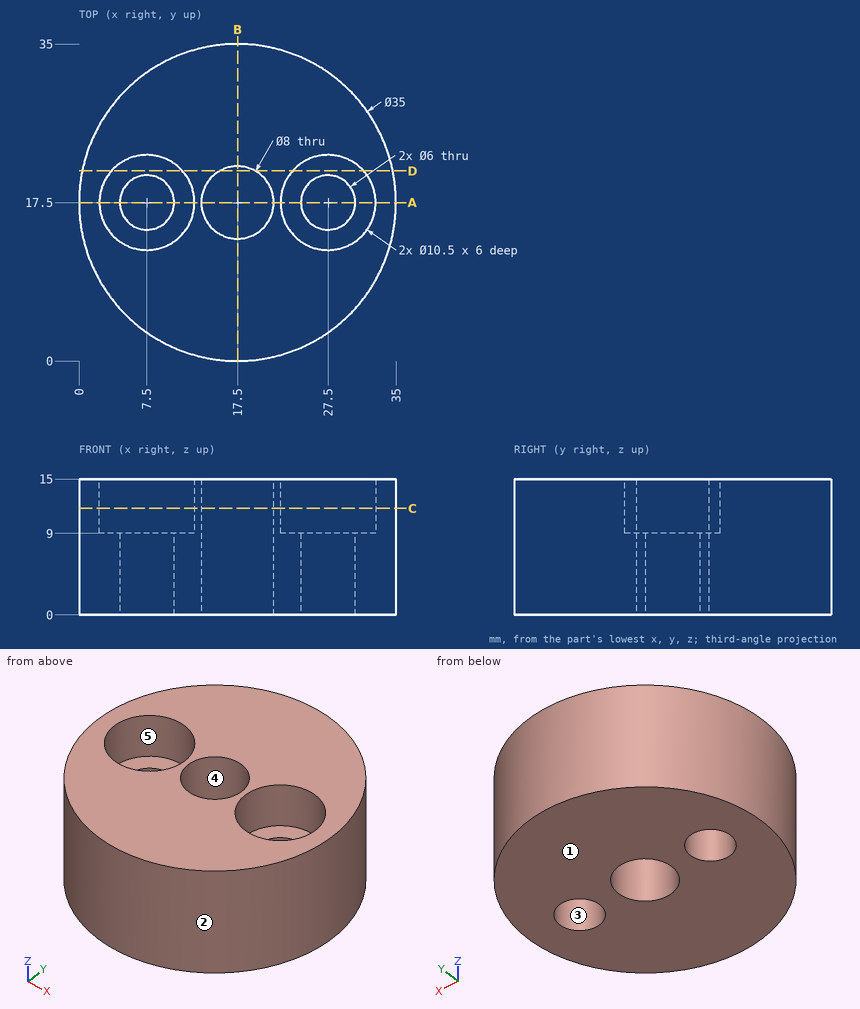
For this review, use the dimensioned drawing (mm, ordinates from the lowest corner) and the shaded views. A direction names the side the tool comes from. Give positions to 0.01 mm unless a question says otherwise; leave off trailing zeros. Order: outer loops, then holes, each group sorted by start corner. A loop starts at its lowest first (then second) coordinate and runs counter-clockwise, first axis right, second up. Notation, with made-up numbers: (6, -24) - (52, -24) arc R20 ccw to (52, 2) - close; hole circle Ø1 at (25, 37.25). An arc over 180 degrees is marked (long way). Use CSV: the item, a comma, the result in double quotes. Start each with the question number.
Q1. We need section B-B, the plane x = 17.5. Write out the cut boundary in (y, z), and give its area (3 significant figures).
Q2. We need section A-A, the plane y = 17.5. Write out the cut boundary in (x, z).
Q3. Tool access review of the marked faces 4 and 5: name each direction out of +Z, -Z, +X, -X, +Y, -Y from which nothing blocks a thin tool from reaching the whole face with its end or side.
Q4. To check wall thickness, follow line 1 along X through (y, z) = (15, 13); line 2 along Z through (x, y) = (24, 14.5); line 3 along Y through (x, z) = (7, 8.5). State the ranges of each line that lie inside material, in increasing order. Write a range as [from, to].
Q5. Clearance check with flat-ended pins moving along their axes: pin 1 Ø8 at (x, y) = (16, 17) entering from -Z; pin 2 Ø8 at (x, y) = (27.5, 17.5) entering from +Z; pin 3 Ø1 at (y, z) = (13.5, 3.5) entering from -X; pin 4 Ø2 at (y, z) = (21.5, 9) entering from -X. State where each tip first meets the part, or that it passes through.
Q6. We need section C-C, the plane z = 11.75. Write out the cut boundary in (x, y).
Q7. We need section D-D, the plane y = 21. Write out the cut boundary in (x, z), and give its area (3 significant figures).
Q8. The part is to be moulded in two halves that separate along Y. For the marked faces 1, 2 and 3, say which applies: +Y half, -Y half, draft (parallel to the pull), parting line (faces both ways), or undercut.
Outcome:
1,outline,"(0, 0) - (13.5, 0) - (13.5, 15) - (0, 15) - close; (21.5, 0) - (35, 0) - (35, 15) - (21.5, 15) - close"
1,area,"405 mm^2"
2,outline,"(0, 0) - (4.5, 0) - (4.5, 9) - (2.25, 9) - (2.25, 15) - (0, 15) - close; (10.5, 0) - (13.5, 0) - (13.5, 15) - (12.75, 15) - (12.75, 9) - (10.5, 9) - close; (21.5, 0) - (24.5, 0) - (24.5, 9) - (22.25, 9) - (22.25, 15) - (21.5, 15) - close; (30.5, 0) - (35, 0) - (35, 15) - (32.75, 15) - (32.75, 9) - (30.5, 9) - close"
3,face 4,"+Z, -Z"
3,face 5,"+Z"
4,line 1,"x = [0.18, 2.88], [12.12, 14.38], [20.62, 22.88], [32.12, 34.82]"
4,line 2,"z = [0, 9]"
4,line 3,"y = [3.5, 14.54], [20.46, 31.5]"
5,pin 1,"stops at z = 0"
5,pin 2,"stops at z = 9"
5,pin 3,"stops at x = 0.35"
5,pin 4,"stops at x = 0.26"
6,outline,"circle Ø35 at (17.5, 17.5); hole circle Ø10.5 at (7.5, 17.5); hole circle Ø8 at (17.5, 17.5); hole circle Ø10.5 at (27.5, 17.5)"
7,outline,"(0.35, 0) - (15.56, 0) - (15.56, 15) - (11.41, 15) - (11.41, 9) - (3.59, 9) - (3.59, 15) - (0.35, 15) - close; (19.44, 0) - (34.65, 0) - (34.65, 15) - (31.41, 15) - (31.41, 9) - (23.59, 9) - (23.59, 15) - (19.44, 15) - close"
7,area,"362 mm^2"
8,face 1,"draft"
8,face 2,"parting line"
8,face 3,"undercut"
